Build history of the part. All positions in model axes, mm. Face numbers are marked on the shaded views. Coordinates: 2 decimals unless noted, no trailing zeros. Order: outer loops, then holes, each group sorted by start corner. A loop starts at its lowest first (then second) coordinate and runs counter-clockwise, first axis right, second up. Notation, with made-up numbers: (5, 39.25) - (17, 39.25) arc R21 cw to (17, 55.25) - close; hole circle Ø1 at (-26.5, 33). An arc over 180 degrees is marked (long way). Return JSON: item names as keys, results as strings.
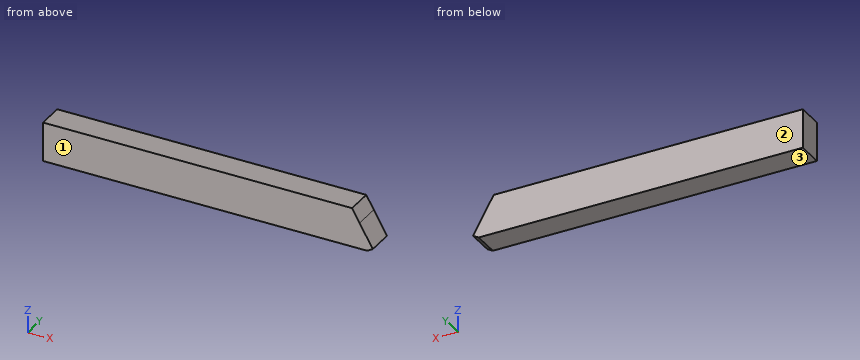
from build123d import *

# Parameters (mm, degrees)
SKETCH1_W               = 25.4
SKETCH1_H               = 25.4
BOSS_EXTRUDE1_DEPTH     = 307.975
BOSS_EXTRUDE2_DEPTH     = 25.4
CUT_EXTRUDE1_DEPTH      = 323.061066955
CUT_EXTRUDE1_DEPTH_BACK = 323.061066955
BOSS_EXTRUDE3_DEPTH     = 25.4


with BuildPart() as part:
    # Sketch1 → Boss-Extrude1 (new body)
    with BuildSketch(Plane(origin=(0, 0, 0), x_dir=(0, 0, -1), z_dir=(1, 0, 0))):
        Rectangle(SKETCH1_W, SKETCH1_H)
    extrude(amount=BOSS_EXTRUDE1_DEPTH)

    # Sketch2 → Boss-Extrude2 (add)
    with BuildSketch(Plane(origin=(0, 12.7, 0), x_dir=(1, 0, 0), z_dir=(0, 1, 0))):
        Polygon((307.975, -12.7), (320.806609733, 9.525), (320.806609733, 12.7), (307.975, 12.7), align=None)
    extrude(amount=-BOSS_EXTRUDE2_DEPTH)

    # Sketch3 → Cut-Extrude1 (cut, two sides: drawn at the far end of the back side and taken through both)
    with BuildSketch(Plane(origin=(0, 12.7, 0), x_dir=(1, 0, 0), z_dir=(0, 1, 0)).offset(-CUT_EXTRUDE1_DEPTH_BACK)):
        Polygon((320.806609733, 9.525), (315.307348419, 12.7), (320.806609733, 12.7), align=None)
    extrude(amount=CUT_EXTRUDE1_DEPTH + CUT_EXTRUDE1_DEPTH_BACK, mode=Mode.SUBTRACT)

    # Sketch4 → Boss-Extrude3 (add)
    with BuildSketch(Plane(origin=(0, 12.7, 0), x_dir=(1, 0, 0), z_dir=(0, 1, 0))):
        Polygon((0, -12.7), (0, -25.4), (300.642651581, -25.4), (307.975, -12.7), align=None)
    extrude(amount=-BOSS_EXTRUDE3_DEPTH)


solid = part.part
1. Cut at B-B on z = 19.5. Give the cut face in (x, y), plus the area to 3 significant figures.
Check values:
{"outline": "(0, -12.7) - (304.05, -12.7) - (304.05, 12.7) - (0, 12.7) - close", "area": "7,720 mm²"}
2. Mould opens along Y. For the marked faces 1, 2 and 3 say: pulls with the +Y half, pulls with the -Y half, needs draft (parallel to the pull), parting line crosses it, or undercut.
Check values:
{"face 1": "pulls with the -Y half", "face 2": "pulls with the +Y half", "face 3": "needs draft"}
3. Cut at A-A on y = 4.25. Give the cut face in (x, z) (3 decimals).
Check values:
{"outline": "(0, -12.7) - (315.307, -12.7) - (320.807, -9.525) - (300.643, 25.4) - (0, 25.4) - close"}
4. Probe L1, parallel to X at y = 10.25, z = 0; L2, parallel to X at y = 6, z = -9.5. List the from-to ranges inside material, lowest first.
Check values:
{"L1": "0 to 315.31", "L2": "0 to 320.79"}
